Verification items for the finished model (mm, model axes). A direction names the side the tool comes from. Coordinates: 2 decimals unless noted, no trailing zeros. Write each loop counter-clockwise with the first axis right and the second up, starting at its lowest first coordinate (ties: lowest second). Pieces come first, ordered by that corner, then holes. Notation, with made-up numbers: (-35.75, 33.25) - (-21.75, 33.25) arc R29 ccw to (-21.75, 56.25) - close; hole circle Ø5 at (-1.75, 42.5). An arc over 180 degrees is marked (long way). Use CSV: the item, a comma, the result in double quotes. Start each with the question number.
```python
from build123d import *

# Parameters (mm, degrees)
CHAMFER1_SIZE      = 1
CHAMFER2_SIZE      = 0.25
FILLET1_R          = 0.5
SKETCH2_R          = 2.5
SKETCH2_R_2        = 3
CUT_EXTRUDE1_DEPTH = 14


with BuildPart() as part:
    # Sketch1 → Revolve1 (revolve)
    with BuildSketch(Plane.XY):
        Polygon((27.5, -12.5), (27.5, -16), (25, -16), (25, -23), (12.4, -23), (12.4, -16), (11.5, -16), (11.5, -5), (0, -5), (0, 0), (24, 0), (24, -12.5), align=None)
    revolve(axis=Axis((0, -394.340972919, 0), (0, 1, 0)))

    # Chamfer1
    chamfer1_edges = [part.edges().sort_by_distance(p)[0] for p in [
        (-12.4, -23, 0),
        (-25, -23, 0),
    ]]
    chamfer(chamfer1_edges, length=CHAMFER1_SIZE)

    # Chamfer2
    chamfer2_edges = [part.edges().sort_by_distance(p)[0] for p in [
        (-11.5, -16, 0),
        (-27.5, -12.5, 0),
        (-27.5, -16, 0),
    ]]
    chamfer(chamfer2_edges, length=CHAMFER2_SIZE)

    # Fillet1
    fillet1_edges = [part.edges().sort_by_distance(p)[0] for p in [
        (-11.5, -5, 0),
        (-24, -12.5, 0),
    ]]
    fillet(fillet1_edges, radius=FILLET1_R)

    # Sketch2 → Cut-Extrude1 (cut)
    with BuildSketch(Plane.XZ.offset(23)):
        with Locations((14.142135624, 14.142135624)):
            Circle(SKETCH2_R)
        with Locations((-14.142135624, 14.142135624)):
            Circle(SKETCH2_R)
        with Locations((14.142135624, -14.142135624)):
            Circle(SKETCH2_R)
        with Locations((-14.142135624, -14.142135624)):
            Circle(SKETCH2_R)
        with Locations((0, 20)):
            Circle(SKETCH2_R_2)
    extrude(amount=-CUT_EXTRUDE1_DEPTH, mode=Mode.SUBTRACT)


solid = part.part
```
Q1. Release check for a two-part mould opening along X. For faces 3 (the flat face through (14, -9, 14)), 4 (the flat face through (10, -23, 10)), 5 (the cylindrical face through (-5.961, -14.271, 26.846)) record: released by +X, released by -X, zero draft, split by the parting line, or undercut.
Q2. Tool access check on faces 1 (the cylindrical face through (13.6, -16.1, 11.7)), 2 (the cylindrical face through (-23.977, -6.084, -1.055)). Record the directions out of +Z, -Z, +X, -X, +Y, -Y that give a thin tool (end or side, any length) a straight path to the whole face; none if there is none.
Q3. Cross-section at B-B (y = -20.5). Record the cut outline in (x, z).
Q4. Scan lines: line 1 along Z through (x, y) = (0, -20.75); line 2 along Z through (x, y) = (-2, -13); line 3 along X through (y, z) = (-13.25, 0). Record each from-to range of solid material in increasing order. Write a range as from..to.
Q5. Cross-section at D-D (y = -13.75). Record the cut outline in (x, z).
Q6. Gauge pin test, flat ends, axial feed: pin 1 (2 mm diameter, centred on y = -20.5, z = 1.5, fed in from +X) (3 decimals); pin 2 (1.5 mm diameter, centred on x = 15, z = 14, fed in from -Y); pin 3 (5 mm diameter, centred on x = -13.5, y = -20, fed in from -Z). Record the tip position at first contact, or that the pin passes through.
Q7. Cross-section at C-C (y = -7). Record the cut outline in (x, z), plus the area to 3 significant figures.
Reply:
1,face 3,"undercut"
1,face 4,"zero draft"
1,face 5,"split by the parting line"
2,face 1,"-Y"
2,face 2,"+Y"
3,outline,"circle Ø50 at (0, 0); hole circle Ø5 at (-14.14, -14.14); hole circle Ø5 at (-14.14, 14.14); hole circle Ø24.8 at (0, 0); hole circle Ø6 at (0, 20); hole circle Ø5 at (14.14, -14.14); hole circle Ø5 at (14.14, 14.14)"
4,line 1,"-25..-12.4, 12.4..17, 23..25"
4,line 2,"-27.43..-11.32, 11.32..17.76, 22.24..27.43"
4,line 3,"-27.5..-11.5, 11.5..27.5"
5,outline,"circle Ø55 at (0, 0); hole circle Ø5 at (-14.14, -14.14); hole circle Ø5 at (-14.14, 14.14); hole circle Ø23 at (0, 0); hole circle Ø6 at (0, 20); hole circle Ø5 at (14.14, -14.14); hole circle Ø5 at (14.14, 14.14)"
6,pin 1,"x = 24.995"
6,pin 2,"y = -9"
6,pin 3,"z = -22.45"
7,outline,"circle Ø48 at (0, 0); hole circle Ø23 at (0, 0)"
7,area,"1,390 mm^2"
